Source: CAD feature listing. Evaluate the final solid. Frame: model axes, mm. A direction names the side the tool comes from. Give positions to 0.01 mm unless a question says otherwise; leave off trailing zeros. Loops run counter-clockwise (first coordinate to the right, second up) from the corner with the lowest first, then second, coordinate; pieces in that order, holes last.
```python
from build123d import *

# Parameters (mm, degrees)
F2_DEPTH = 51
F3_DEPTH = 1.2
F5_DEPTH = 5
F6_DEPTH = 5


with BuildPart() as f2:
    # F1 (on Top) → F2 (new body)
    with BuildSketch(Plane.XY):
        with BuildLine():
            ThreePointArc((11.909081537, 0), (13.6518289963, 13.6518289963), (0, 11.909081537))
            ThreePointArc((0, 11.909081537), (-13.6518289963, 13.6518289963), (-11.909081537, 0))
            ThreePointArc((-11.909081537, 0), (-13.6518289963, -13.6518289963), (0, -11.909081537))
            ThreePointArc((0, -11.909081537), (13.6518289963, -13.6518289963), (11.909081537, 0))
        make_face()
        with BuildLine():
            ThreePointArc((0.1948051948, 9.1982723157), (12.8033008589, 12.8033008589), (9.1982723157, 0.1948051948))
            ThreePointArc((9.1982723157, 0.1948051948), (9.0435595774, 0), (9.1982723157, -0.1948051948))
            ThreePointArc((9.1982723157, -0.1948051948), (12.8033008589, -12.8033008589), (0.1948051948, -9.1982723157))
            ThreePointArc((0.1948051948, -9.1982723157), (0, -9.0435595774), (-0.1948051948, -9.1982723157))
            ThreePointArc((-0.1948051948, -9.1982723157), (-12.8033008589, -12.8033008589), (-9.1982723157, -0.1948051948))
            ThreePointArc((-9.1982723157, -0.1948051948), (-9.0435595774, 0), (-9.1982723157, 0.1948051948))
            ThreePointArc((-9.1982723157, 0.1948051948), (-12.8033008589, 12.8033008589), (-0.1948051948, 9.1982723157))
            ThreePointArc((-0.1948051948, 9.1982723157), (0, 9.0435595774), (0.1948051948, 9.1982723157))
        make_face(mode=Mode.SUBTRACT)
    extrude(amount=F2_DEPTH)

    # F1 (on Top) → F3 (join)
    with BuildSketch(Plane.XY):
        with BuildLine():
            ThreePointArc((9.1982723157, -0.1948051948), (9.0435595774, 0), (9.1982723157, 0.1948051948))
            ThreePointArc((9.1982723157, 0.1948051948), (12.8033008589, 12.8033008589), (0.1948051948, 9.1982723157))
            ThreePointArc((0.1948051948, 9.1982723157), (0, 9.0435595774), (-0.1948051948, 9.1982723157))
            ThreePointArc((-0.1948051948, 9.1982723157), (-12.8033008589, 12.8033008589), (-9.1982723157, 0.1948051948))
            ThreePointArc((-9.1982723157, 0.1948051948), (-9.0435595774, 0), (-9.1982723157, -0.1948051948))
            ThreePointArc((-9.1982723157, -0.1948051948), (-12.8033008589, -12.8033008589), (-0.1948051948, -9.1982723157))
            ThreePointArc((-0.1948051948, -9.1982723157), (0, -9.0435595774), (0.1948051948, -9.1982723157))
            ThreePointArc((0.1948051948, -9.1982723157), (12.8033008589, -12.8033008589), (9.1982723157, -0.1948051948))
        make_face()
    extrude(amount=F3_DEPTH)

    # F4 (on face) → F5 (join)
    with BuildSketch(Plane.XY.offset(51)):
        with BuildLine():
            ThreePointArc((-11.909081537, 0), (-14.3440182045, 2.1288348735), (-15.8330666624, 5))
            Line((-15.8330666624, 5), (-22.0820734114, 5))
            Line((-22.0820734114, 5), (-22.0820734114, -5))
            Line((-22.0820734114, -5), (-15.8330666624, -5))
            ThreePointArc((-15.8330666624, -5), (-14.3440182045, -2.1288348735), (-11.909081537, 0))
        make_face()
    extrude(amount=-F5_DEPTH)

    # F4 (on face) → F6 (join)
    with BuildSketch(Plane.XY.offset(51)):
        with BuildLine():
            Line((15, -3.090918463), (15, 3.090918463))
            ThreePointArc((15, 3.090918463), (13.6518289963, 1.3481710037), (11.909081537, 0))
            ThreePointArc((11.909081537, 0), (13.6518289963, -1.3481710037), (15, -3.090918463))
        make_face()
    extrude(amount=-F6_DEPTH)


solid = f2.part
```
(1) Mould query, pull axis Y, two halves, no side actions, for faces 1 (the flat face through (14, 0, 46)), 2 (the cylindrical face through (13.8, 13.5, 25.1)), 3 (the flat face through (-22.082, 0, 49)). Classes: pulls with the +Y half, pulls with the -Y half, needs draft (parallel to the pull), parting line crosses it, or undercut.
A:
face 1: undercut
face 2: undercut
face 3: needs draft
(2) Ray query, line 1 along Y through (x, z) = (7.5, 26.5); line 2 along X through (y, z) = (10.5, 9.5). Return the intervals inside material, ascending.
A:
line 1: y = -16.2 to -15, 15 to 16.2
line 2: x = -15.67 to -14.37, -0.63 to 0.63, 14.37 to 15.67
(3) Section C-C, the plane z = 6.5. Return the cut outline in (x, y).
A:
outline: (-11.91, 0) arc R8.7 ccw (long way) to (0, -11.91) arc R8.7 ccw (long way) to (11.91, 0) arc R8.7 ccw (long way) to (0, 11.91) arc R8.7 ccw (long way) to start; hole (-9.2, -0.19) arc R7.5 ccw (long way) to (-0.19, -9.2) arc R0.2 cw to (0.19, -9.2) arc R7.5 ccw (long way) to (9.2, -0.19) arc R0.2 cw to (9.2, 0.19) arc R7.5 ccw (long way) to (0.19, 9.2) arc R0.2 cw to (-0.19, 9.2) arc R7.5 ccw (long way) to (-9.2, 0.19) arc R0.2 cw to start
(4) First-contact query: pin 1 (2.5 mm diameter, centred on x = -20, z = 48.5, fed in from -Y); pin 2 (10 mm diameter, centred on y = -10.5, z = 14, fed in from -X); pin 3 (1 mm diameter, centred on x = -11.5, z = 43.5, fed in from +Y). Flat tips, straight axial feed; report the tip coordinate or a pass-through.
A:
pin 1: stops at y = -5
pin 2: stops at x = -16.2
pin 3: stops at y = 15.46
(5) Section D-D, the plane x = 14. Return the cut outline in (y, z).
A:
outline: (-13.28, 0) - (-1.72, 0) - (-1.72, 46) - (1.72, 46) - (1.72, 0) - (13.28, 0) - (13.28, 51) - (11.24, 51) - (11.24, 1.2) - (3.76, 1.2) - (3.76, 51) - (-3.76, 51) - (-3.76, 1.2) - (-11.24, 1.2) - (-11.24, 51) - (-13.28, 51) - close
(6) Section A-A, the plane y = 7.5. Return the cut outline in (x, z).
A:
outline: (-16.2, 0) - (16.2, 0) - (16.2, 51) - (15, 51) - (15, 1.2) - (-15, 1.2) - (-15, 51) - (-16.2, 51) - close
(7) Reachability of faces 4 (the flat face through (-18, 0, 46)), 5 (the flat face through (15, 0, 49)), 6 (the cylindrical face through (-12.6, -13, 25.8)) from +Z, -Z, +X, -X, +Y, -Y: full face, straight path, thin tool, end or side. Return the list, or none.
A:
face 4: -Z, -X
face 5: +Z, -Z, +X
face 6: +Z
